```python
from build123d import *

# Parameters (mm, degrees)
BOSS_EXTRUDE1_DEPTH = 6
SHELL1_T            = -1
FILLET1_R           = 1


with BuildPart() as part:
    # Sketch1 → Boss-Extrude1 (new body)
    with BuildSketch(Plane(origin=(0, 0, 0), x_dir=(1, 0, 0), z_dir=(0, 1, 0))):
        with BuildLine():
            Line((0, 0), (10.57, 0))
            Line((10.57, 0), (10.57, -30))
            Line((10.57, -30), (0, -30))
            ThreePointArc((0, -30), (2.434164903, -15), (0, 0))
        make_face()
    extrude(amount=BOSS_EXTRUDE1_DEPTH)

    # Shell1
    shell1_openings = [part.faces().sort_by_distance(p)[0] for p in [
        (6.071410828, 0, 15),
        (2.434164903, 3, 15),
    ]]
    offset(amount=SHELL1_T, openings=shell1_openings, kind=Kind.INTERSECTION)

    # Fillet1
    fillet1_edges = [part.edges().sort_by_distance(p)[0] for p in [
        (10.57, 6, 15),
        (5.285, 6, 0),
        (10.57, 3, 0),
        (10.57, 3, 30),
        (5.285, 6, 30),
    ]]
    fillet(fillet1_edges, radius=FILLET1_R)


solid = part.part
```
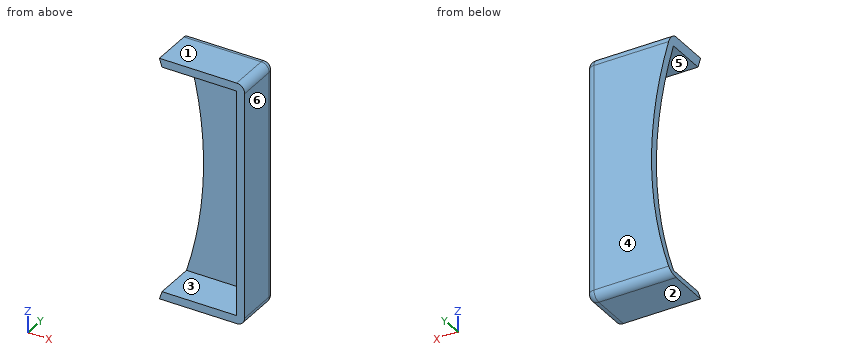
Design review of the part built by this model. Coordinates are the model's own, in mm. Face numbers are marked on the shaded views. A direction names the side the tool comes from. Give positions to 0.01 mm unless a question says otherwise; leave off trailing zeros. Write each loop counter-clockwise with the first axis right and the second up, starting at its lowest first coordinate (ties: lowest second). Pieces come first, ordered by that corner, then holes. Notation, with made-up numbers: (37, 2.25) -> (66, 2.25) arc R19 cw to (66, 10.25) -> close; hole circle Ø10 at (86, 43.25). An arc over 180 degrees is marked (long way). Answer in a Markdown table with one row per item.
(1) Consider section B-B (y = 1.75). State the section outline as (x, z) points, then the cut area to 3 significant figures.
Results:
| item | result |
|---|---|
| outline | (0, 0) -> (9.57, 0) arc R1 ccw to (10.57, 1) -> (10.57, 29) arc R1 ccw to (9.57, 30) -> (0, 30) arc R47.43 cw to (0.32, 29) -> (9.57, 29) -> (9.57, 1) -> (0.32, 1) arc R47.43 cw to start |
| area | 48.4 mm2 |
(2) To check wall thickness, follow probe 1 along Z at (x, y) = (8.75, 3.75); probe 2 along X at (y, z) = (1.25, 14.5); probe 3 along Y at (x, z) = (2.25, 24.5). State the ranges of each line that lie inside material, in increasing order.
Results:
| item | result |
|---|---|
| probe 1 | 0 to 1, 29 to 30 |
| probe 2 | 9.57 to 10.57 |
| probe 3 | 5 to 6 |
(3) Clearance check with flat-ended pins moving along their axes: pin 1 (4 mm diameter, centred on x = 9.5, z = 25, fed in from -Y); pin 2 (1.5 mm diameter, centred on x = 4.5, z = 14, fed in from -Y). State where each tip first meets the part, or that it passes through.
Results:
| item | result |
|---|---|
| pin 1 | y = 0 |
| pin 2 | y = 5 |
(4) Consider section A-A (x = 4.25). State the section outline as (y, z) points, then the cut area to 3 significant figures.
Results:
| item | result |
|---|---|
| outline | (0, 0) -> (5, 0) arc R1 ccw to (6, 1) -> (6, 29) arc R1 ccw to (5, 30) -> (0, 30) -> (0, 29) -> (5, 29) -> (5, 1) -> (0, 1) -> close |
| area | 39.6 mm2 |
(5) Consider section D-D (z = 16.5). State the section outline as (x, y) points.
Results:
| item | result |
|---|---|
| outline | (2.41, 5) -> (9.57, 5) -> (9.57, 0) -> (10.57, 0) -> (10.57, 5) arc R1 ccw to (9.57, 6) -> (2.41, 6) -> close |
(6) Consider section C-C (x = 1.5). State the section outline as (y, z) points.
Results:
| item | result |
|---|---|
| outline | (0, 0) -> (5, 0) arc R1 ccw to (6, 1) -> (6, 5.63) -> (5, 5.63) -> (5, 1) -> (0, 1) -> close; (0, 29) -> (5, 29) -> (5, 24.37) -> (6, 24.37) -> (6, 29) arc R1 ccw to (5, 30) -> (0, 30) -> close |
(7) For the marked faces 5 and 6, list the 3-axis set-ups (+Z, -Z, +X, -X, +Y, -Y) from which the entire face can be reached by the end or side of a thin tool; tool diameter is ignored.
Results:
| item | result |
|---|---|
| face 5 | -X, -Y |
| face 6 | +Z, -Z, +X, +Y, -Y |
(8) Mouldability with a two-part tool opening along Z and no side actions: class the marked faces 1, 2, 3 and 4 as +Z half, -Z half, draft (parallel to the pull), parting line (faces both ways), or undercut.
Results:
| item | result |
|---|---|
| face 1 | +Z half |
| face 2 | -Z half |
| face 3 | undercut |
| face 4 | draft |
